For this review, take the finished solid that the model builds, in its own axes (mm). A direction names the side the tool comes from. Coordinates: 2 decimals unless noted, no trailing zeros. Order: outer loops, then holes, each group sorted by start corner. A loop starts at its lowest first (then second) coordinate and runs counter-clockwise, first axis right, second up. Notation, with made-up numbers: M 80.25,30.5 L 89.25,30.5 A22 ccw 89.25,56.5 Z; hole C 47,6.5 d2. An arc over 180 degrees is marked long. Use one line per item in the form item = value. Start each with the question number.
```python
from build123d import *

# Parameters (mm, degrees)
SKETCH1_R           = 10.1
BOSS_EXTRUDE1_DEPTH = 3
BOSS_EXTRUDE2_DEPTH = 49
SKETCH3_R           = 10.1
SKETCH3_R_2         = 2.5
BOSS_EXTRUDE3_DEPTH = 3
BOSS_EXTRUDE6_DEPTH = 3
SKETCH5_R           = 1.75
BOSS_EXTRUDE7_DEPTH = 5


with BuildPart() as part:
    # Sketch1 → Boss-Extrude1 (new body)
    with BuildSketch(Plane(origin=(0, 0, 0), x_dir=(1, 0, 0), z_dir=(0, 1, 0))):
        with Locations(Location((0, 0, 0), (0, 0, 270))):
            Circle(SKETCH1_R)
    extrude(amount=BOSS_EXTRUDE1_DEPTH)

    # Sketch2 → Boss-Extrude2 (add)
    with BuildSketch(Plane(origin=(0, 3, 0), x_dir=(1, 0, 0), z_dir=(0, 1, 0))):
        with BuildLine():
            Line((-2.952954218, 9.658678035), (-2.338973638, 7.650438048))
            ThreePointArc((-2.338973638, 7.650438048), (0, 8), (2.338973638, 7.650438048))
            Line((2.338973638, 7.650438048), (2.952954218, 9.658678035))
            ThreePointArc((2.952954218, 9.658678035), (0, 10.1), (-2.952954218, 9.658678035))
        make_face()
        with BuildLine():
            Line((9.658678035, 2.952954218), (7.650438048, 2.338973638))
            ThreePointArc((7.650438048, 2.338973638), (8, 0), (7.650438048, -2.338973638))
            Line((7.650438048, -2.338973638), (9.658678035, -2.952954218))
            ThreePointArc((9.658678035, -2.952954218), (10.1, 0), (9.658678035, 2.952954218))
        make_face()
        with BuildLine():
            Line((2.952954218, -9.658678035), (2.338973638, -7.650438048))
            ThreePointArc((2.338973638, -7.650438048), (0, -8), (-2.338973638, -7.650438048))
            Line((-2.338973638, -7.650438048), (-2.952954218, -9.658678035))
            ThreePointArc((-2.952954218, -9.658678035), (0, -10.1), (2.952954218, -9.658678035))
        make_face()
        with BuildLine():
            Line((-9.658678035, -2.952954218), (-7.650438048, -2.338973638))
            ThreePointArc((-7.650438048, -2.338973638), (-8, 0), (-7.650438048, 2.338973638))
            Line((-7.650438048, 2.338973638), (-9.658678035, 2.952954218))
            ThreePointArc((-9.658678035, 2.952954218), (-10.1, 0), (-9.658678035, -2.952954218))
        make_face()
    extrude(amount=BOSS_EXTRUDE2_DEPTH)

    # Sketch3 → Boss-Extrude3 (add)
    with BuildSketch(Plane(origin=(0, 52, 0), x_dir=(1, 0, 0), z_dir=(0, 1, 0))):
        with Locations(Location((0, 0, 0), (0, 0, 270))):
            Circle(SKETCH3_R)
        with Locations(Location((0, 0, 0), (0, 0, 270))):
            Circle(SKETCH3_R_2, mode=Mode.SUBTRACT)
    extrude(amount=BOSS_EXTRUDE3_DEPTH)

    # Sketch4 → Boss-Extrude6 (add)
    with BuildSketch(Plane.XZ):
        with BuildLine():
            Line((-11.532649592, 5.999832781), (-4, 36.31))
            ThreePointArc((-4, 36.31), (0, 40.31), (4, 36.31))
            Line((4, 36.31), (11.532649592, 5.999832781))
            ThreePointArc((11.532649592, 5.999832781), (0, -13), (-11.532649592, 5.999832781))
        make_face()
    extrude(amount=BOSS_EXTRUDE6_DEPTH)

    # Sketch5 → Boss-Extrude7 (add)
    with BuildSketch(Plane(origin=(0, 0, 0), x_dir=(1, 0, 0), z_dir=(0, 1, 0))):
        with Locations(Location((0, -36.31, 0), (0, 0, 90))):
            Circle(SKETCH5_R)
    extrude(amount=BOSS_EXTRUDE7_DEPTH)


solid = part.part
```
1. Consider section C-C, the plane x = -6.75. Write out the cut boundary in (y, z).
2. Tool access review of faces 4 (the flat face through (0, 5, 36)), 5 (the flat face through (8.67, 27.16, -2.65)), 6 (the flat face through (-2.64, 27.16, 8.64)), 7 (the cylindrical face through (-8, 27, 0)): name each direction out of +Z, -Z, +X, -X, +Y, -Y from which nothing blocks a thin tool from reaching the whole face with its end or side.
3. The part is to be moulded in two halves that separate along Y. For faces 1 (the flat face through (-8.67, 27.16, 2.65)), 2 (the flat face through (-2, 55, 2)), 3 (the flat face through (-7.82, -1.48, 20.94)), say which applies: pulls with the +Y half, pulls with the -Y half, needs draft (parallel to the pull), parting line crosses it, or undercut.
4. To check wall thickness, follow line 1 (X direction, y = 53.4, z = 0); line 2 (Y direction, x = -3.5, z = -4.5); line 3 (Y direction, x = 7, z = -10). State the ranges of each line that lie inside material, in increasing order.
5. For pin 1 Ø8 at (x, y) = (-8, 14) entering from +Z; pin 2 Ø5 at (x, y) = (5, 28.5) entering from -Z; pin 3 Ø1 at (x, z) = (10, 18) entering from -Y; pin 4 Ø1.8 at (x, z) = (0.5, 36) entering from +Y, all flat-tipped, find the tip position at first contact; note any pin that passes through.
6. Consider section B-B, the plane z = 4.5. Write out the cut boundary in (x, y).
7. Consider section A-A, the plane y = 30. Write out the cut boundary in (x, z).
8. Consider section D-D, the plane y = 1.5. Write out the cut boundary in (x, z), plus the area to 3 significant figures.
Answers follow:
q1.outline = M -3,-11.11 L 0,-11.11 L 0,-7.51 L 3,-7.51 L 3,7.51 L 0,7.51 L 0,25.24 L -3,25.24 Z; M 52,-7.51 L 55,-7.51 L 55,7.51 L 52,7.51 Z
q2.face_4 = +Z, +X, -X, +Y
q2.face_5 = -Z
q2.face_6 = -X
q2.face_7 = none
q3.face_1 = undercut
q3.face_2 = pulls with the +Y half
q3.face_3 = needs draft
q4.line_1 = -10.1 to -2.5, 2.5 to 10.1
q4.line_2 = -3 to 3, 52 to 55
q4.line_3 = -3 to 0
q5.pin_1 = 2.95
q5.pin_2 = -9.79
q5.pin_3 = through
q5.pin_4 = 5
q6.outline = M -12.2,-3 L 12.2,-3 L 12.2,0 L 9.04,0 L 9.04,3 L -9.04,3 L -9.04,0 L -12.2,0 Z; M -9.04,52 L 9.04,52 L 9.04,55 L -9.04,55 Z
q7.outline = M -9.66,-2.95 L -7.65,-2.34 A8 cw -7.65,2.34 L -9.66,2.95 A10.1 ccw Z; M -2.95,-9.66 A10.1 ccw 2.95,-9.66 L 2.34,-7.65 A8 cw -2.34,-7.65 Z; M -2.95,9.66 L -2.34,7.65 A8 cw 2.34,7.65 L 2.95,9.66 A10.1 ccw Z; M 7.65,-2.34 L 9.66,-2.95 A10.1 ccw 9.66,2.95 L 7.65,2.34 A8 cw Z
q8.outline = C 0,0 d20.2; C 0,36.31 d3.5
q8.area = 330 mm²
